Geometry: see drawing. Coordinates: mm, zero at the bounding-box minimum. Round coordinates to 2 decimals unless told otherwise and drop trailing zeros. Order: outer loops, then holes, each group sorted by start corner. A loop starts at its lowest first (then second) coordinate and runs counter-clockwise, first axis right, second up. Notation, with made-up numbers: (-32.75, 32.5) -> (-16.75, 32.5) arc R15 ccw to (-16.75, 43.5) -> close; hole circle Ø9 at (41, 32). An arc over 180 degrees is marked (long way). Put each result on its own line as item: value.
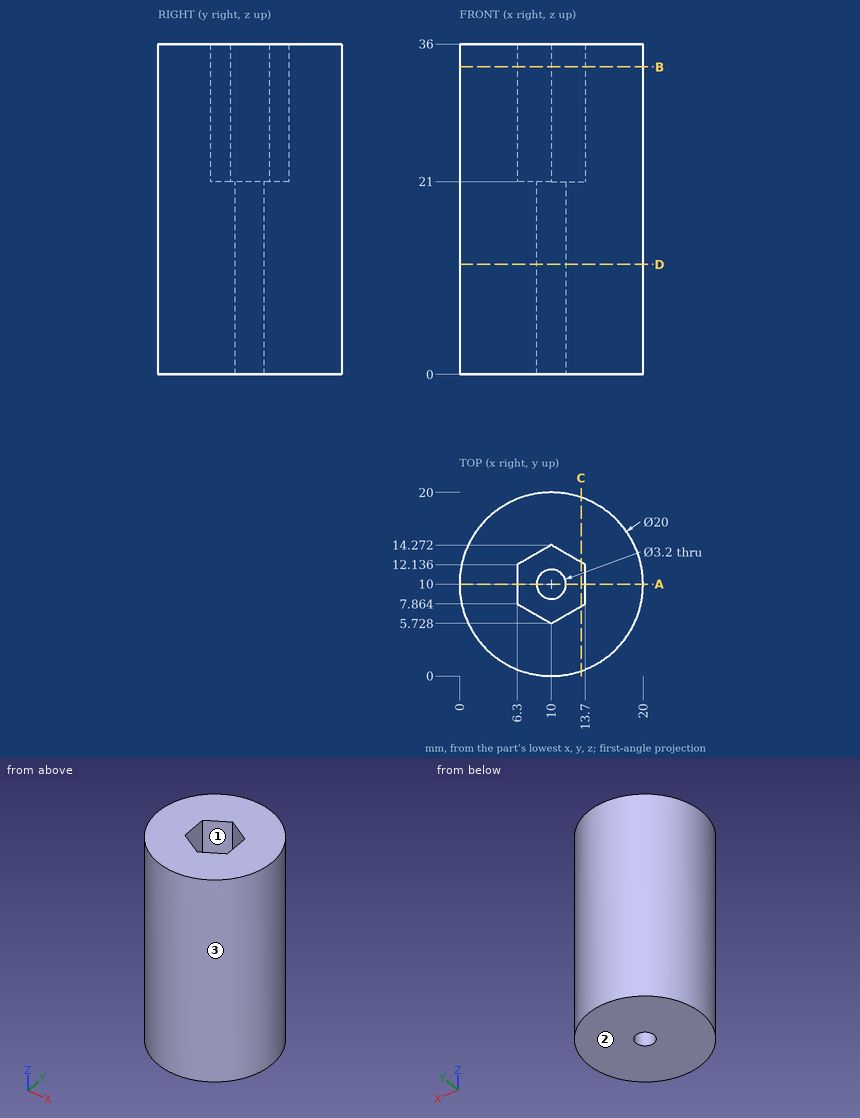
1. Contact query for flat-ended pins moving along their axis: P1, Ø2, axis at x = 11, y = 2.5, coming from the -Z side; P2, Ø1.3, axis at y = 9, z = 29, coming from the -X side; P3, Ø3, axis at x = 16, z = 17, coming from the +Y side; P4, Ø2, axis at x = 7.5, z = 31, coming from the +Y side. Output: stop coordinate, or through.
Ans:
P1: z = 0
P2: x = 0.01
P3: y = 18.93
P4: y = 19.89
2. Cut plane A-A on y = 10. Return loops of the section in (x, z), and give its area (3 significant figures).
Ans:
outline: (0, 0) -> (8.4, 0) -> (8.4, 21) -> (6.3, 21) -> (6.3, 36) -> (0, 36) -> close; (11.6, 0) -> (20, 0) -> (20, 36) -> (13.7, 36) -> (13.7, 21) -> (11.6, 21) -> close
area: 542 mm²
3. Cut plane C-C on x = 13.25. Return loops of the section in (y, z).
Ans:
outline: (0.54, 0) -> (19.46, 0) -> (19.46, 36) -> (12.4, 36) -> (12.4, 21) -> (7.6, 21) -> (7.6, 36) -> (0.54, 36) -> close
4. Draft query along Y for the marked faces 1, 2 and 3. Return one class per face: +Y half, -Y half, draft (parallel to the pull), parting line (faces both ways), or undercut.
Ans:
face 1: undercut
face 2: draft
face 3: parting line
5. Cut plane D-D on z = 12. Return loops of the section in (x, y), and give its area (3 significant figures).
Ans:
outline: circle Ø20 at (10, 10); hole circle Ø3.2 at (10, 10)
area: 306 mm²
6. Material intervals for probe 1 along Y at (x, z) = (10, 4.75); probe 2 along Z at (x, y) = (9.5, 6.25); probe 3 along Y at (x, z) = (8.5, 34) (1 decimal), sorted ascending.
Ans:
probe 1: 0 to 8.4, 11.6 to 20
probe 2: 0 to 21
probe 3: 0.1 to 6.6, 13.4 to 19.9
7. Cut plane B-B on z = 33.5. Return loops of the section in (x, y).
Ans:
outline: circle Ø20 at (10, 10); hole (6.3, 7.86) -> (10, 5.73) -> (13.7, 7.86) -> (13.7, 12.14) -> (10, 14.27) -> (6.3, 12.14) -> close
